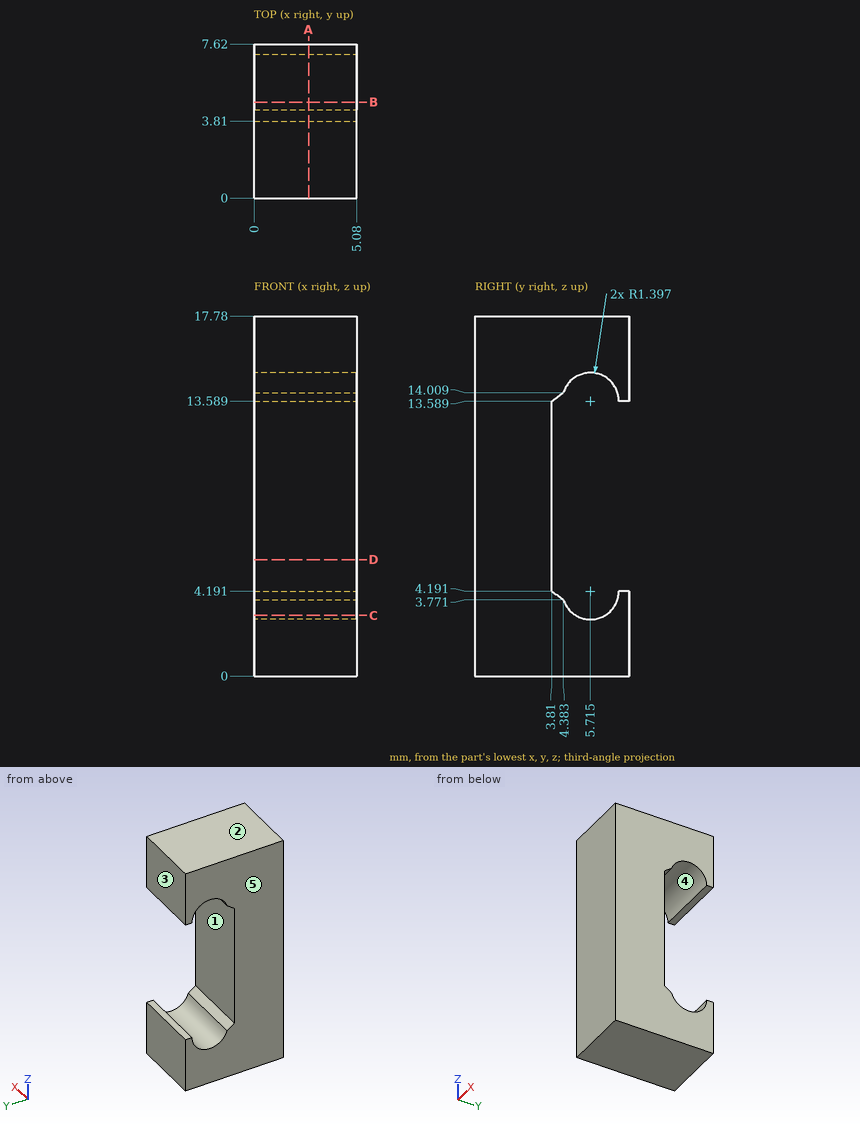
Could you check a few things on this drawing? It's one solid part, dimensions in mm from its lowest x, y, z. A direction names the side the tool comes from. Give positions to 0.01 mm unless a question says otherwise; leave off trailing zeros. Order: outer loops, then holes, each group sorted by start corner. A loop starts at its lowest first (then second) coordinate and runs counter-clockwise, first axis right, second up. Notation, with made-up numbers: (-16.5, 62.5) - (-3.5, 62.5) arc R26 ccw to (-3.5, 86.5) - close; hole circle Ø11 at (-9, 89). An arc over 180 degrees is marked (long way). Answer as a JSON object with one key per item and string values. Group by question number.
Item 1: If we mould it in two halves opening along Z, with no side actions, what happens to the marked faces 1, 2 and 3? For each: pulls with the +Z half, pulls with the -Z half, needs draft (parallel to the pull), parting line crosses it, or undercut.
Item 2: Which directions (+Z, -Z, +X, -X, +Y, -Y) give clear straight access to the entire face, cutting with the end or side of a thin tool? Please do the marked faces 4 and 5.
Item 3: For P1, Ø3, axis at x = 3, y = 1.5, coming from the -Z side, with a flat end and sliding along its axis, tell me the tip position at first contact or that it passes through.
Item 4: If we section it at C-C on z = 3: Please give me the cut outline in (x, y) (1 decimal), and give its area (3 significant figures).
Item 5: If we section it at D-D on z = 5.75: Please give me the cut outline in (x, y).
Item 6: Please list where these lines run through material, in increasing order: probe 1 along Y at (x, z) = (1.4, 9.5); probe 2 along Z at (x, y) = (1.8, 5); probe 3 along Z at (x, y) = (0.85, 4).
Item 7: If we section it at A-A on x = 2.7: Please give me the cut outline in (y, z) (1 decimal).
Item 8: If we section it at B-B on y = 4.75: Please give me the cut outline in (x, z).
Result set:
{
 "1": {"face 1": "undercut", "face 2": "pulls with the +Z half", "face 3": "needs draft"},
 "2": {"face 4": "+X, -X", "face 5": "+Z, -Z, -X, +Y, -Y"},
 "3": {"P1": "z = 0"},
 "4": {"outline": "(0, 0) - (5.1, 0) - (5.1, 5) - (0, 5) - close; (0, 6.4) - (5.1, 6.4) - (5.1, 7.6) - (0, 7.6) - close", "area": "31.3 mm²"},
 "5": {"outline": "(0, 0) - (5.08, 0) - (5.08, 3.81) - (0, 3.81) - close"},
 "6": {"probe 1": "0 to 3.81", "probe 2": "0 to 2.99, 14.79 to 17.78", "probe 3": "0 to 4.05, 13.73 to 17.78"},
 "7": {"outline": "(0, 0) - (7.6, 0) - (7.6, 4.2) - (7.1, 4.2) arc R1.4 cw to (4.4, 3.8) - (3.8, 4.2) - (3.8, 13.6) - (4.4, 14) arc R1.4 cw to (7.1, 13.6) - (7.6, 13.6) - (7.6, 17.8) - (0, 17.8) - close"},
 "8": {"outline": "(0, 0) - (5.08, 0) - (5.08, 3.18) - (0, 3.18) - close; (0, 14.6) - (5.08, 14.6) - (5.08, 17.78) - (0, 17.78) - close"}
}
